```python
from build123d import *

# Parameters (mm, degrees)
SKETCH1_R               = 51.1048
SKETCH1_R_2             = 49.53
BOSS_EXTRUDE1_DEPTH     = 50.8
CUT_SWEEP1_START        = -51.104800053
CUT_SWEEP1_OUTLINE_R    = 2.749999961
CUT_SWEEP1_DEPTH        = 1.651201698
MIRROR2_START           = -51.104800053
MIRROR2_COPY_1_SKETCH_R = 2.749999961
MIRROR2_COPY_1_DEPTH    = 1.651201698
SKETCH18_R              = 2.749999961
SKETCH18_W              = 10.000000066
SKETCH18_H              = 6.99999997
CUT_EXTRUDE1_DEPTH      = 89.340484472
SKETCH18_3_R            = 2.749999961
SKETCH18_3_W            = 10.000000066
SKETCH18_3_H            = 6.99999997
CUT_EXTRUDE2_DEPTH      = 89.340484472


# Read off the part's stored shape, not the designer's step: Cut-Sweep1
with BuildPart() as part:
    # Sketch1 → Boss-Extrude1 (new, symmetric)
    with BuildSketch(Plane(origin=(0, 0, 0), x_dir=(1, 0, 0), z_dir=(0, 1, 0))):
        with Locations(Location((0, 0, 0), (0, 0, 270))):
            Circle(SKETCH1_R)
        with Locations(Location((0, 0, 0), (0, 0, 270))):
            Circle(SKETCH1_R_2, mode=Mode.SUBTRACT)
    extrude(amount=BOSS_EXTRUDE1_DEPTH, both=True)

    # Cut-Sweep1 outline → Cut-Sweep1 (cut)
    with BuildSketch(Plane(origin=(0, 0, 0), x_dir=(0.9940563382223202, 0, -0.10886687485195803), z_dir=(0.10886687485195805, 0, 0.9940563382223203)).offset(CUT_SWEEP1_START)):
        Circle(CUT_SWEEP1_OUTLINE_R)
    cut_sweep1 = extrude(amount=CUT_SWEEP1_DEPTH, mode=Mode.SUBTRACT)

    # Mirror1: Cut-Sweep1 across plane
    add(cut_sweep1.mirror(Plane(origin=(0, 0, 0), x_dir=(0, 0, 1), z_dir=(1, 0, 0))), mode=Mode.SUBTRACT)

    # Mirror2: Cut-Sweep1 across plane
    add(cut_sweep1.mirror(Plane.XY), mode=Mode.SUBTRACT)

    # Mirror2 copy 1 sketch → Mirror2 copy 1 (cut)
    with BuildSketch(Plane(origin=(0, 0, 0), x_dir=(-0.9940563382223202, 0, 0.10886687485195803), z_dir=(-0.10886687485195805, 0, -0.9940563382223203)).offset(MIRROR2_START)):
        Circle(MIRROR2_COPY_1_SKETCH_R)
    extrude(amount=MIRROR2_COPY_1_DEPTH, mode=Mode.SUBTRACT)

    # Sketch18 → Cut-Extrude1 (cut, through all)
    with BuildSketch(Plane.XY):
        with Locations(Location((0, 3.81, 0), (0, 0, 90))):
            Circle(SKETCH18_R)
        with Locations((0, -8.579999985)):
            Rectangle(SKETCH18_W, SKETCH18_H)
    extrude(amount=-CUT_EXTRUDE1_DEPTH, mode=Mode.SUBTRACT)

    # Sketch18<3> → Cut-Extrude2 (cut, through all)
    with BuildSketch(Plane.XY):
        with Locations(Location((0, -3.81, 0), (0, 0, 89.999999966))):
            Circle(SKETCH18_3_R)
        with Locations((0, 8.579999985)):
            Rectangle(SKETCH18_3_W, SKETCH18_3_H)
    extrude(amount=CUT_EXTRUDE2_DEPTH, mode=Mode.SUBTRACT)


solid = part.part
```
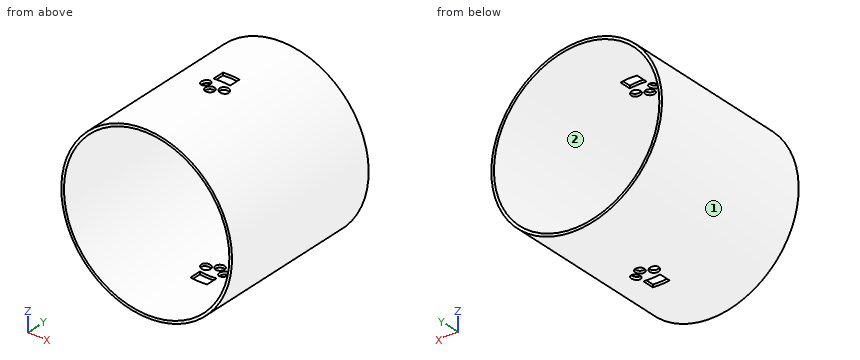
Part model, mm, in its own coordinate system. Face numbers are marked on the shaded views. Round coordinates to 2 decimals unless told otherwise and drop trailing zeros. Write each loop counter-clockwise with the first axis right and the second up, starting at its lowest first coordinate (ties: lowest second). Pieces come first, ordered by that corner, then holes.
Item 1: Cut at C-C, the plane x = -29.5. Give the cut face in (y, z), plus the area to 3 significant figures.
Results:
outline: (-50.8, -41.73) - (50.8, -41.73) - (50.8, -39.79) - (-50.8, -39.79) - close; (-50.8, 39.79) - (50.8, 39.79) - (50.8, 41.73) - (-50.8, 41.73) - close
area: 395 mm2
Item 2: Cut at D-D, the plane y = 23. Give the cut face in (x, z), plus the area to 3 significant figures.
Results:
outline: circle Ø102.21 at (0, 0); hole circle Ø99.06 at (0, 0)
area: 498 mm2
Item 3: Cut at B-B, the plane x = 0. Give the cut face in (y, z).
Results:
outline: (-50.8, -51.1) - (-12.08, -51.1) - (-12.08, -49.53) - (-50.8, -49.53) - close; (-50.8, 49.53) - (-6.56, 49.53) - (-6.56, 51.1) - (-50.8, 51.1) - close; (-5.08, -51.1) - (1.06, -51.1) - (1.06, -49.53) - (-5.08, -49.53) - close; (-1.06, 49.53) - (5.08, 49.53) - (5.08, 51.1) - (-1.06, 51.1) - close; (6.56, -51.1) - (50.8, -51.1) - (50.8, -49.53) - (6.56, -49.53) - close; (12.08, 49.53) - (50.8, 49.53) - (50.8, 51.1) - (12.08, 51.1) - close
Item 4: Drop flat-ended pins along their axis: pin 1 Ø1.5 at (y, z) = (-27, 31.5) entering from -X; pin 2 Ø1 at (x, y) = (-37.5, 38.5) entering from +Z; pin 3 Ø10 at (y, z) = (31.5, -22.5) entering from -X. Give the stop position or say it passes through.
Results:
pin 1: stops at x = -40.82
pin 2: stops at z = 35.25
pin 3: stops at x = -48.02
Item 5: Two-plate mould, pull along X, no slides. Class the marked faces 1 and 2: +X half, -X half, draft (parallel to the pull), parting line (faces both ways), or undercut.
Results:
face 1: parting line
face 2: undercut
Item 6: Probe L1, parallel to X at y = -0.5, z = 41; L2, parallel to X at y = -3.5, z = -11; L3, parallel to Z at x = 18.5, y = -8.5. List the from-to ranges inside material, lowest first.
Results:
L1: x = -30.51 to -27.79, 27.79 to 30.51
L2: x = -49.91 to -48.29, 48.29 to 49.91
L3: z = -47.64 to -45.95, 45.95 to 47.64
Item 7: Cut at A-A, the plane z = 0. Give the cut face in (x, y), plus the area to 3 significant figures.
Results:
outline: (-51.1, -50.8) - (-49.53, -50.8) - (-49.53, 50.8) - (-51.1, 50.8) - close; (49.53, -50.8) - (51.1, -50.8) - (51.1, 50.8) - (49.53, 50.8) - close
area: 320 mm2
